Could you check a few things on this model? Use its own coordinates, in mm. A direction names the side the tool comes from. Give positions to 0.01 mm unless a question says otherwise; leave off trailing zeros. Write each loop counter-clockwise with the first axis right and the second up, starting at its lowest first coordinate (ties: lowest second). Pieces come first, ordered by that corner, then holes. Notation, with made-up numbers: (-15, 74) -> (15, 74) arc R23 cw to (15, 104) -> close; hole circle Ø11 at (61.25, 69). An arc over 180 degrees is marked (long way). One line per question, with ' | ' between items.
from build123d import *

# Parameters (mm, degrees)
F3_R           = 4
F4_DEPTH       = 25
F6_D           = 5.1
F6_DEPTH       = 6.4
F6_CSINK_D     = 6.12
F6_CSINK_ANGLE = 90
F6_TIP         = 1.5321945785
F7_D           = 5.1
F7_DEPTH       = 6.4
F7_CSINK_D     = 6.12
F7_CSINK_ANGLE = 90
F7_TIP         = 1.5321945785


with BuildPart() as f4:
    # F3 (on Top) → F4 (new body)
    with BuildSketch(Plane.XY):
        Circle(F3_R)
    extrude(amount=F4_DEPTH)

    # F6
    with Locations(Plane.XY.offset(25)):
        with Locations((0, 0)):
            CounterSinkHole(F6_D / 2, F6_CSINK_D / 2, depth=F6_DEPTH, counter_sink_angle=F6_CSINK_ANGLE)
            with Locations((0, 0, -(F6_DEPTH + F6_TIP / 2))):  # 118° drill point
                Cone(0, F6_D / 2, F6_TIP, mode=Mode.SUBTRACT)

    # F7
    with Locations(Plane(origin=(0, 0, 0), x_dir=(1, 0, 0), z_dir=(0, 0, -1))):
        with Locations((0, 0)):
            CounterSinkHole(F7_D / 2, F7_CSINK_D / 2, depth=F7_DEPTH, counter_sink_angle=F7_CSINK_ANGLE)
            with Locations((0, 0, -(F7_DEPTH + F7_TIP / 2))):  # 118° drill point
                Cone(0, F7_D / 2, F7_TIP, mode=Mode.SUBTRACT)


solid = f4.part
Q1. On a 3-axis mill with a long thin cutter (end or side, diameter ignored), from which of +Z, -Z, +X, -X, +Y, -Y can I reach the whole of each face in a straight line? I mean faces 1 (the cylindrical face through (-1.18, -2.26, 21.5)), 2 (the cylindrical face through (-1.18, 2.26, 3.5)). Say none if no direction works.
Answer below:
face 1: +Z | face 2: -Z
Q2. Imagine slicing it at A-A on z = 23.25. Please give me the cut outline in (x, y), and give its area (3 significant figures).
Answer below:
outline: circle Ø8 at (0, 0); hole circle Ø5.1 at (0, 0) | area: 29.8 mm^2
Q3. If I drill on line 1 along Y through (x, z) = (0, 4.55); line 2 along X through (y, z) = (-1.75, 21); line 3 along X through (y, z) = (1, 22.75), over which ranges is the centre line in solid material (lowest first)?
Answer below:
line 1: y = -4 to -2.55, 2.55 to 4 | line 2: x = -3.6 to -1.85, 1.85 to 3.6 | line 3: x = -3.87 to -2.35, 2.35 to 3.87
Q4. Imagine slicing it at C-C on z = 7.5. Please give me the cut outline in (x, y).
Answer below:
outline: circle Ø8 at (0, 0); hole circle Ø1.44 at (0, 0)
Q5. If we mould it in two halves opening along X, with no side actions, what happens to faces 3 (the conical face through (0.42, 0.13, 17.33)), 4 (the cylindrical face through (-0.867, -3.905, 12.325))? For each: +X half, -X half, draft (parallel to the pull), parting line (faces both ways), or undercut.
Answer below:
face 3: undercut | face 4: parting line
Q6. Will these pins go through, and if not, where does the flat tip stop? pin 1 (4.5 mm diameter, centred on x = 0, y = 0, fed in from -Z); pin 2 (1 mm diameter, centred on y = -1, z = 19, fed in from +X); pin 3 (1 mm diameter, centred on x = -2, y = -1, fed in from -Z).
Answer below:
pin 1: stops at z = 6.58 | pin 2: stops at x = 3.97 | pin 3: stops at z = 0.32
Q7. Imagine slicing it at B-B on z = 10. Please give me the cut outline in (x, y).
Answer below:
outline: circle Ø8 at (0, 0)
